Geometry check sheet. Reference: the model listing, model coordinates, mm. A direction names the side the tool comes from. Coordinates: 2 decimals unless noted, no trailing zeros. Loops run counter-clockwise (first coordinate to the right, second up) from the corner with the lowest first, then second, coordinate; pieces in that order, holes last.
from build123d import *

# Parameters (mm, degrees)
SKETCH1_R               = 2.5
BOSS_EXTRUDE1_DEPTH     = 12.5
CUT_EXTRUDE1_DEPTH      = 38.91437722
CUT_EXTRUDE1_DEPTH_BACK = 38.91437722
SKETCH2_W               = 10
SKETCH2_H               = 5
F_6_0MM_DOWEL_HOLE1_D   = 6


with BuildPart() as part:
    # Sketch1 → Boss-Extrude1 (new, symmetric)
    with BuildSketch(Plane(origin=(0, 0, 0), x_dir=(1, 0, 0), z_dir=(0, 1, 0))):
        with BuildLine():
            Line((-10, 10), (-5, 10))
            Line((-5, 10), (-5, -10))
            Line((-5, -10), (-10, -10))
            ThreePointArc((-10, -10), (-15, -15), (-10, -20))
            Line((-10, -20), (-5, -20))
            Line((-5, -20), (-5, -32.5))
            Line((-5, -32.5), (0, -32.5))
            Line((0, -32.5), (0, 32.5))
            Line((0, 32.5), (-5, 32.5))
            Line((-5, 32.5), (-5, 20))
            Line((-5, 20), (-10, 20))
            ThreePointArc((-10, 20), (-15, 15), (-10, 10))
        make_face()
        with Locations(Location((-10, 15, 0), (0, 0, 270))):
            Circle(SKETCH1_R, mode=Mode.SUBTRACT)
        with Locations(Location((-10, -15, 0), (0, 0, 270))):
            Circle(SKETCH1_R, mode=Mode.SUBTRACT)
    extrude(amount=BOSS_EXTRUDE1_DEPTH, both=True)

    # Sketch2 → Cut-Extrude1 (cut, two sides: drawn at the far end of the back side and taken through both)
    with BuildSketch(Plane.XY.offset(-CUT_EXTRUDE1_DEPTH_BACK)):
        with Locations((-10, 10)):
            Rectangle(SKETCH2_W, SKETCH2_H)
        with Locations((-10, -10)):
            Rectangle(SKETCH2_W, SKETCH2_H)
    extrude(amount=CUT_EXTRUDE1_DEPTH + CUT_EXTRUDE1_DEPTH_BACK, mode=Mode.SUBTRACT)

    # Ø6.0mm Dowel Hole1 (through all)
    with Locations(Plane(origin=(0, 0, 0), x_dir=(0, 0, -1), z_dir=(1, 0, 0))):
        with Locations((0, 0)):
            Hole(F_6_0MM_DOWEL_HOLE1_D / 2)


solid = part.part
1) Depth check by flat-ended pin: pin 1 (8 mm diameter, centred on x = -12.5, z = 13.5, fed in from -Y); pin 2 (12.5 mm diameter, centred on y = 5.5, z = 15.5, fed in from -X); pin 3 (1.5 mm diameter, centred on x = -8.5, y = 2.5, fed in from +Z); pin 4 (3 mm diameter, centred on x = -8.5, z = -17, fed in from +Y). Enter the tip coordinate at first touch or a pass-through.
Data:
pin 1: stops at y = -7.5
pin 2: stops at x = -15
pin 3: stops at z = 20
pin 4: stops at y = 7.5
2) Section check D-D on y = -10.5. Record the cut outline in (x, z), and give its area (3 significant figures).
Data:
outline: (-5, -32.5) - (0, -32.5) - (0, 32.5) - (-5, 32.5) - close
area: 325 mm2
3) Mould release check, pull along Y, two halves, no side actions. Record for faces 1 (the flat face through (-7, -7.5, 15)), 2 (the flat face through (-3, 12.5, 0)), 3 (the flat face through (-7, 0, -20)), 4 (the cylindrical face through (-3, 0, -3)): +Y half, -Y half, draft (parallel to the pull), parting line (faces both ways), or undercut.
Data:
face 1: -Y half
face 2: +Y half
face 3: draft
face 4: undercut
4) Section check A-A on x = -6. Record the cut outline in (y, z).
Data:
outline: (-7.5, -20) - (7.5, -20) - (7.5, -10) - (-7.5, -10) - close; (-7.5, 10) - (7.5, 10) - (7.5, 20) - (-7.5, 20) - close
5) Access from +Z, -Z, +X, -X, +Y, -Y to the whole of each face (thin tool, end or side, straight path). Record for faces 5 (the flat face through (-8, 0, -10)), 6 (the flat face through (-7, -7.5, -15)), 7 (the flat face through (-8, 0, 20)), 8 (the flat face through (-7, 7.5, 15)).
Data:
face 5: -X, +Y, -Y
face 6: +Z, -Z, -X, -Y
face 7: +Z, -X, +Y, -Y
face 8: +Z, -Z, -X, +Y
6) Material ranges on probe 1 along Z at (x, y) = (-10.25, 3); probe 2 along Z at (x, y) = (-6, -1.5); probe 3 along Z at (x, y) = (-9.5, -4), recorded low to high.
Data:
probe 1: z = -19.99 to -17.49, -12.51 to -10.01, 10.01 to 12.51, 17.49 to 19.99
probe 2: z = -20 to -10, 10 to 20
probe 3: z = -20 to -17.45, -12.55 to -10, 10 to 12.55, 17.45 to 20
7) Section check B-B on z = 0. Record the cut outline in (x, y).
Data:
outline: (-5, -12.5) - (0, -12.5) - (0, -3) - (-5, -3) - close; (-5, 3) - (0, 3) - (0, 12.5) - (-5, 12.5) - close
8) Section check C-C on z = -15. Record the cut outline in (x, y).
Data:
outline: (-15, -7.5) - (-12.5, -7.5) - (-12.5, 7.5) - (-15, 7.5) - close; (-7.5, -7.5) - (-5, -7.5) - (-5, -12.5) - (0, -12.5) - (0, 12.5) - (-5, 12.5) - (-5, 7.5) - (-7.5, 7.5) - close
